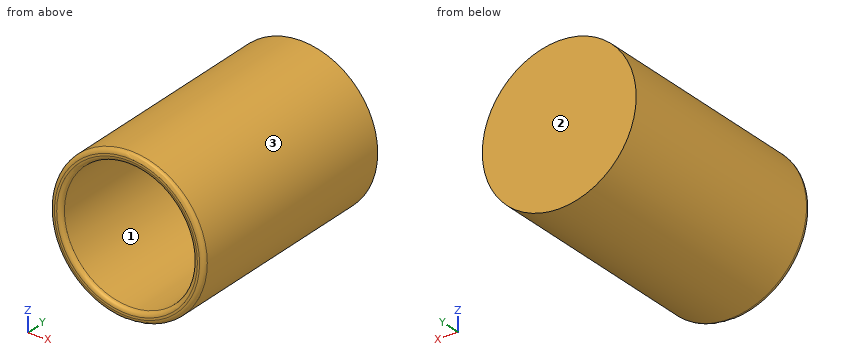
from build123d import *

# Parameters (mm, degrees)
F1_DEPTH    = 123.825
F2_DEPTH    = 25.4
F1_FACE_R   = 44.45
F1_FACE_R_2 = 38.1
F3_DEPTH    = 9.525
F4_R        = 2.54


with BuildPart() as f1:
    # F0 (on Front) → F1 (new body)
    with BuildSketch(Plane.XZ):
        with BuildLine():
            ThreePointArc((44.45, 0), (0, 44.45), (-44.45, 0))
            ThreePointArc((-44.45, 0), (0, -44.45), (44.45, 0))
        make_face()
        with BuildLine():
            ThreePointArc((-38.1, 0), (0, 38.1), (38.1, 0))
            ThreePointArc((38.1, 0), (0, -38.1), (-38.1, 0))
        make_face(mode=Mode.SUBTRACT)
    extrude(amount=F1_DEPTH)

    # F0 (on Front) → F2 (join)
    with BuildSketch(Plane.XZ):
        with BuildLine():
            ThreePointArc((44.45, 0), (0, 44.45), (-44.45, 0))
            ThreePointArc((-44.45, 0), (0, -44.45), (44.45, 0))
        make_face()
        with BuildLine():
            ThreePointArc((-38.1, 0), (0, 38.1), (38.1, 0))
            ThreePointArc((38.1, 0), (0, -38.1), (-38.1, 0))
        make_face(mode=Mode.SUBTRACT)
    extrude(amount=F2_DEPTH)

    # F0 (on Front) + F1_face (on face) → F3 (join)
    with BuildSketch(Plane.XZ):
        with BuildLine():
            ThreePointArc((-38.1, 0), (0, -38.1), (38.1, 0))
            ThreePointArc((38.1, 0), (0, 38.1), (-38.1, 0))
        make_face()
    with BuildSketch(Plane.XZ.offset(123.825)):
        Circle(F1_FACE_R)
        Circle(F1_FACE_R_2, mode=Mode.SUBTRACT)
    extrude(amount=F3_DEPTH)

    # F4
    f4_edges = [f1.edges().sort_by_distance(p)[0] for p in [
        (-44.45, -133.35, 0),
        (-38.1, -133.35, 0),
    ]]
    fillet(f4_edges, radius=F4_R)


solid = f1.part
Can you work these out from the model? Positions are in its coordinate system, mm. Face numbers are marked on the shaded views. Coordinates: 2 decimals unless noted, no trailing zeros. Write each loop counter-clockwise with the first axis right and the second up, starting at its lowest first coordinate (ties: lowest second). Pieces come first, ordered by that corner, then holes. Notation, with made-up numbers: (70.5, -21) -> (83.5, -21) arc R31 ccw to (83.5, 10) -> close; hole circle Ø10 at (9.25, 88). An arc over 180 degrees is marked (long way). Write each question's results on one line, items separated by ' | '. Start each with the question number.
Q1. Imagine slicing it at A-A (x = 0). Write out the boundary of the cut face in (y, z) (3 decimals), then the cut area to 3 significant figures.
Q2. If I drill on probe 1 along X at (y, z) = (-100.5, -1); probe 2 along Z at (x, y) = (0, -76); probe 3 along Y at (x, z) = (7, 6) (3 decimals), over which ranges is the centre line in solid material (lowest first)?
Q3. I'm going to push flat-ended pins straight in: pin 1 (3 mm diameter, centred on y = -86, z = -13, fed in from +X); pin 2 (1 mm diameter, centred on y = -115.5, z = 29, fed in from -X); pin 3 (2 mm diameter, centred on x = -6.5, z = 28, fed in from -Y) (3 decimals). Where does each tip first touch, or does it pass through?
Q4. We'd pull the mould along X, two halves only. Please class the marked faces 1, 2 and 3: +X half, -X half, draft (parallel to the pull), parting line (faces both ways), or undercut.
Q5. Imagine slicing it at C-C (y = -27). Write out the boundary of the cut face in (x, z), then the cut area to 3 significant figures.
Q6. Imagine slicing it at B-B (z = 0). Write out the boundary of the cut face in (x, y) (3 decimals), then the cut area to 3 significant figures.
Taken from the geometry:
1) outline: (-133.35, -41.91) arc R2.54 ccw to (-130.81, -44.45) -> (0, -44.45) -> (0, 44.45) -> (-130.81, 44.45) arc R2.54 ccw to (-133.35, 41.91) -> (-133.35, 40.64) arc R2.54 ccw to (-130.81, 38.1) -> (-9.525, 38.1) -> (-9.525, -38.1) -> (-130.81, -38.1) arc R2.54 ccw to (-133.35, -40.64) -> close | area: 2,410 mm^2
2) probe 1: x = -44.44 to -38.09, 38.09 to 44.44 | probe 2: z = -44.45 to -38.1, 38.1 to 44.45 | probe 3: y = -9.525 to 0
3) pin 1: stops at x = 42.94 | pin 2: stops at x = -34.11 | pin 3: stops at y = -9.525
4) face 1: undercut | face 2: draft | face 3: parting line
5) outline: circle Ø88.9 at (0, 0); hole circle Ø76.2 at (0, 0) | area: 1,650 mm^2
6) outline: (-44.45, -130.81) arc R2.54 ccw to (-41.91, -133.35) -> (-40.64, -133.35) arc R2.54 ccw to (-38.1, -130.81) -> (-38.1, -9.525) -> (38.1, -9.525) -> (38.1, -130.81) arc R2.54 ccw to (40.64, -133.35) -> (41.91, -133.35) arc R2.54 ccw to (44.45, -130.81) -> (44.45, 0) -> (-44.45, 0) -> close | area: 2,410 mm^2
